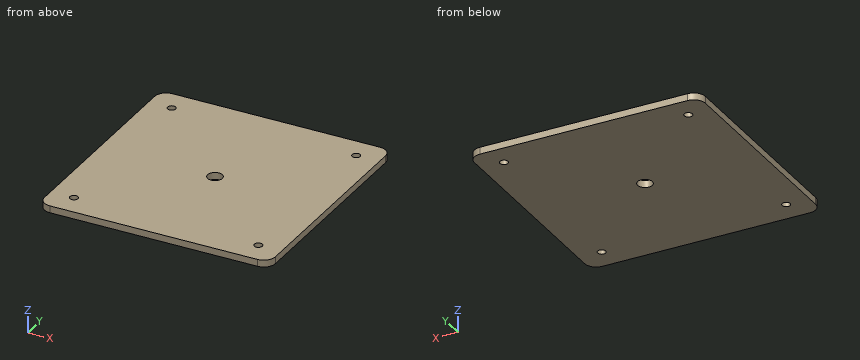
Autodesk Fusion 360 part; units mm, degrees
sketch "Sketch1" plane through (0, 0, 0) normal (0, 0, 1) x (1, 0, 0)
  line L0 (0, 0) -> (100, 0)
  line L1 (100, 0) -> (100, 100)
  line L2 (100, 100) -> (0, 100)
  line L3 (0, 100) -> (0, 0)
  dimension "d1" = 100
  dimension "d2" = 100
extrude "Extrude1" add sketch "Sketch1" along normal blind 5
sketch "Sketch2" plane through (0, 0, 5) normal (0, 0, 1) x (-1, 0, 0)
  line L0 (0, -100) -> (0, 0)
  line L1 (0, 0) -> (-100, 0)
  line L2 (-100, 0) -> (-100, -100)
  line L3 (-100, -100) -> (0, -100)
  line L4 (-15, -15) -> (-85, -15)
  line L5 (-85, -15) -> (-85, -85)
  line L6 (-85, -85) -> (-15, -85)
  line L7 (-15, -85) -> (-15, -15)
  line L8 (-15, -85) -> (-10.0503, -89.9497)
  line L9 (-15, -85) -> (-8, -85) construction
  line L10 (-85, -85) -> (-89.9497, -89.9497)
  line L11 (-85, -85) -> (-78, -85) construction
  line L12 (-15, -15) -> (-10.0503, -10.0503)
  line L13 (-15, -15) -> (-8, -15) construction
  line L14 (-85, -15) -> (-89.9497, -10.0503)
  line L15 (-85, -15) -> (-78, -15) construction
  dimension "d5" = 45
  dimension "d6" = 7
  dimension "d7" = 135
  dimension "d8" = 7
  dimension "d9" = 7
  dimension "d10" = 45
  dimension "d11" = 135
  dimension "d12" = 7
extrude "Extrude2" cut sketch "Sketch2" against normal blind 2 contours L0 L1 L2 L3 | L4 L5 L6 L7
hole "Hole1" at (89.9497, 89.9497, 5) direction (0, 0, -1) diameter 3 depth 67 tip angle 118
hole "Hole2" at (10.0503, 89.9497, 5) direction (0, 0, -1) diameter 3 depth 4.7 tip angle 118
hole "Hole3" at (10.0503, 10.0503, 5) at (89.9497, 10.0503, 5) direction (0, 0, -1) diameter 3 depth 4.7 tip angle 118
hole "Hole4" at (50, 50, 3) direction (0, 0, -1) diameter 6.4 depth 5 tip angle 180
hole "Hole5" at (10.0503, 89.9497, 3) direction (0, 0, -1) diameter 3 depth 5 tip angle 180
hole "Hole6" at (10.0503, 10.0503, 3) direction (0, 0, -1) diameter 3 depth 5 tip angle 180
hole "Hole7" at (89.9497, 10.0503, 3) direction (0, 0, -1) diameter 3 depth 5 tip angle 180
fillet "Fillet1" radius 5 4 edges at (0, 0, 1.5) (100, 0, 1.5) (100, 100, 1.5) (0, 100, 1.5)
hole "Hole8" at (10.0503, 89.9497, 5) at (89.9497, 89.9497, 5) at (10.0503, 10.0503, 5) at (89.9497, 10.0503, 5) direction (0, 0, -1) diameter 3.5 depth 100 tip angle 180
The listing builds one solid part. Answer for the finished solid, in the listing's coordinates (mm). Give positions to 0.01 mm unless a question says otherwise; leave off trailing zeros. Order: outer loops, then holes, each group sorted by start corner. A loop starts at its lowest first (then second) coordinate and runs counter-clockwise, first axis right, second up. Notation, with made-up numbers: (-28, 86.5) -> (16, 86.5) arc R21 cw to (16, 123.5) -> close; hole circle Ø2 at (43, 36). An arc over 180 degrees is marked (long way). One line per item, written item: value.
1) A flat-ended cylindrical pin translates along its axis: P1, Ø1, axis at x = 45, y = 71.5, coming from the -Z side. Find the tip coordinate at first contact, or state that the pin passes through.
Reported:
P1: stops at z = 0
2) Find the intervals of material crossed by line 1 (Y direction, x = 50, z = 2); line 2 (X direction, y = 90, z = 0.9), in increasing order.
Reported:
line 1: y = 0 to 46.8, 53.2 to 100
line 2: x = 0 to 8.3, 11.8 to 88.2, 91.7 to 100
3) Find section A-A, the plane x = 50. Determine the outline of the cut face in (y, z), plus the area to 3 significant figures.
Reported:
outline: (0, 0) -> (46.8, 0) -> (46.8, 3) -> (0, 3) -> close; (53.2, 0) -> (100, 0) -> (100, 3) -> (53.2, 3) -> close
area: 281 mm^2
